Can you work these out from the model? Positions are in its coordinate system, mm. Face numbers are marked on the shaded views. Round coordinates to 2 decimals unless told otherwise and drop trailing zeros. Order: outer loops, then holes, each group sorted by start corner. A loop starts at its lowest first (then second) coordinate and runs counter-clockwise, first axis right, second up.
from build123d import *

# Parameters (mm, degrees)
F0_R     = 30
F0_R_2   = 22
F1_DEPTH = 50
F2_SIZE  = 0.5
F3_SIZE  = 0.5


with BuildPart() as f1:
    # F0 (on Top) → F1 (new body)
    with BuildSketch(Plane.XY):
        Circle(F0_R)
        Circle(F0_R_2, mode=Mode.SUBTRACT)
    extrude(amount=F1_DEPTH)

    # F2
    f2_edges = [f1.edges().sort_by_distance(p)[0] for p in [
        (-30, 0, 50),
    ]]
    chamfer(f2_edges, length=F2_SIZE)

    # F3
    f3_edges = [f1.edges().sort_by_distance(p)[0] for p in [
        (-22, 0, 50),
    ]]
    chamfer(f3_edges, length=F3_SIZE)


solid = f1.part
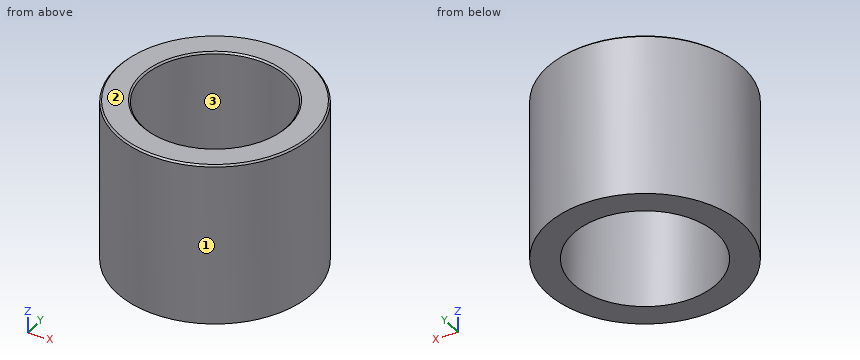
(1) I want a section at A-A, the plane x = 0. List the corners of the cut face in (y, z) for me.
(2) I'm going to push flat-ended pins straight in: pin 1 Ø12 at (x, z) = (12, 43) entering from +Y; pin 2 Ø5 at (y, z) = (-22.5, 43) entering from +X; pin 3 Ø6 at (x, z) = (-20, 28) entering from +Y. Where does each tip first touch, or does it pass through?
(3) Please list where these lines run through material, in increasing order: probe 1 along X at (y, z) = (-0.5, 8.5); probe 2 along Y at (x, z) = (0, 30.5); probe 3 along X at (y, z) = (-4, 18.5).
(4) If we mould it in two halves opening along X, with no side actions, what happens to the marked faces 1, 2 and 3? For each: pulls with the +X half, pulls with the -X half, needs draft (parallel to the pull), parting line crosses it, or undercut.
(5) I want a section at C-C, the plane z = 47. List the corners of the cut face in (x, y) for me.
Ans:
1. outline: (-30, 0) - (-22, 0) - (-22, 49.5) - (-22.5, 50) - (-29.5, 50) - (-30, 49.5) - close; (22, 0) - (30, 0) - (30, 49.5) - (29.5, 50) - (22.5, 50) - (22, 49.5) - close
2. pin 1: stops at y = 29.39
2. pin 2: stops at x = 22.36
2. pin 3: stops at y = 24.72
3. probe 1: x = -30 to -21.99, 21.99 to 30
3. probe 2: y = -30 to -22, 22 to 30
3. probe 3: x = -29.73 to -21.63, 21.63 to 29.73
4. face 1: parting line crosses it
4. face 2: needs draft
4. face 3: undercut
5. outline: circle Ø60 at (0, 0); hole circle Ø44 at (0, 0)
